```python
from build123d import *

# Parameters (mm, degrees)
F0_R            = 11
F1_DEPTH        = 7
F1_COPIES_COUNT = 3


# Not quite as in the source:
# - a pattern or mirror of a feature is missing from the dataset's text; its kind, count and spacing are read off the source's solid


with BuildPart() as f1:
    # F0 (on Top) → F1 (new body)
    with BuildSketch(Plane.XY):
        with BuildLine():
            ThreePointArc((0, 11), (7.7781745931, 7.7781745931), (11, 0))
            ThreePointArc((11, 0), (7.7781745931, -7.7781745931), (0, -11))
            Line((0, -11), (0, -18.5))
            Line((0, -18.5), (26, -18.5))
            ThreePointArc((26, -18.5), (42.0452305564, -1.25), (26, 16))
            Line((26, 16), (0, 16))
            Line((0, 16), (0, 11))
        make_face()
        with Locations((26, 0)):
            Circle(F0_R, mode=Mode.SUBTRACT)
    extrude(amount=F1_DEPTH)

    # F1_copies: F1 ×3 about axis
    f1_copies_axis = Axis((0, 0, 0), (0, 0, 1))


with BuildPart() as f1_1:
    add(f1.part)
    for i in range(1, F1_COPIES_COUNT):
        add(f1.part.rotate(f1_copies_axis, i * 360 / F1_COPIES_COUNT))


solid = f1_1.part
```
CAD build for the part. Positions are in the model's coordinates, mm. A direction names the side the tool comes from. Round coordinates to 2 decimals unless told otherwise and drop trailing zeros. Write each loop counter-clockwise with the first axis right and the second up, starting at its lowest first coordinate (ties: lowest second). Pieces come first, ordered by that corner, then holes. Notation, with made-up numbers: (7, -4) -> (58, -4) arc R23 cw to (58, 11) -> close; hole circle Ø9 at (61, -6). An arc over 180 degrees is marked (long way). Answer in a Markdown table with one row per item. Add a question column.
Item 1: Drill centre lines: line 1 (Y direction, x = 26, z = 2.5); line 2 (Y direction, x = -13, z = 3.5); line 3 (X direction, y = 3.5, z = 1.25). Where is each one in solid material? Low to high. Write a range as from..to.
Item 2: Mould opens along X. For faces 6 (the face through (42.04, -1.61, 3.45)), 7 (the face through (-11, -6, 7)), 8 (the face through (-21.107, -15.082, 3.451)) say: pulls with the +X half, pulls with the -X half, needs draft (parallel to the pull), parting line crosses it, or undercut.
Item 3: Drop flat-ended pins along their axis: pin 1 Ø2 at (x, z) = (17, 3.5) entering from -Y; pin 2 Ø3 at (y, z) = (2.5, 2) entering from +X; pin 3 Ø3.5 at (x, z) = (20.5, 3) entering from +Y. Give the stop position or say it passes through.
Item 4: Saw through at D-D, the plane z = 1. Write the cut outline in (x, y).
Item 5: Which spindle directions (+Z, -Z, +X, -X, +Y, -Y) get a long thin tool onto all of the face, cutting with end or side? Do faces 1 (the face through (19, 16, 3)), 2 (the face through (-23.436, 8.592, 3.451)), 3 (the face through (-11, -6, 0)), 4 (the face through (36.161, -4.213, 3.451)), 5 (the face through (17, -18.5, 3)). Say none if no direction does.
Item 6: Saw through at B-B, the plane y = 6.5. Write the cut outline in (x, z).
Item 7: Saw through at C-C, the plane x = -13. Write the cut outline in (y, z), then the cut area to 3 significant figures.
Item 8: Saw through at A-A, the plane x = 34. Write the cut outline in (y, z).
Findings below:
| question | item | result |
|---|---|---|
| 1 | line 1 | y = -18.5..-11, 11..16 |
| 1 | line 2 | y = -38.1..-33.52, -11.52..11.52, 33.52..39.27 |
| 1 | line 3 | x = -20.5..-10.43, 10.43..15.57, 36.43..41.38 |
| 2 | face 6 | pulls with the +X half |
| 2 | face 7 | needs draft |
| 2 | face 8 | undercut |
| 3 | pin 1 | stops at y = -18.5 |
| 3 | pin 2 | stops at x = 41.9 |
| 3 | pin 3 | stops at y = 16 |
| 4 | outline | (-29.02, -13.27) arc R17.3 ccw to (0.86, -30.52) -> (7.79, -18.5) -> (26, -18.5) arc R17.3 ccw to (26, 16) -> (12.12, 16) -> (3.02, 31.77) arc R17.3 ccw to (-26.86, 14.52) -> (-19.92, 2.5) -> close; hole circle Ø22 at (-13, -22.52); hole circle Ø22 at (-13, 22.52); hole circle Ø22 at (0, 0); hole circle Ø22 at (26, 0) |
| 5 | face 1 | +Z, -Z, +X, +Y |
| 5 | face 2 | +Z, -Z, -X |
| 5 | face 3 | -Z, +X, -X, +Y, -Y |
| 5 | face 4 | +Z, -Z |
| 5 | face 5 | +Z, -Z, +X, -Y |
| 6 | outline | (-22.23, 0) -> (-8.87, 0) -> (-8.87, 7) -> (-22.23, 7) -> close; (8.87, 0) -> (17.13, 0) -> (17.13, 7) -> (8.87, 7) -> close; (34.87, 0) -> (40.21, 0) -> (40.21, 7) -> (34.87, 7) -> close |
| 7 | outline | (-38.1, 0) -> (-33.52, 0) -> (-33.52, 7) -> (-38.1, 7) -> close; (-11.52, 0) -> (11.52, 0) -> (11.52, 7) -> (-11.52, 7) -> close; (33.52, 0) -> (39.27, 0) -> (39.27, 7) -> (33.52, 7) -> close |
| 7 | area | 234 mm^2 |
| 8 | outline | (-15.86, 0) -> (-7.55, 0) -> (-7.55, 7) -> (-15.86, 7) -> close; (7.55, 0) -> (13.36, 0) -> (13.36, 7) -> (7.55, 7) -> close |
